For this review, use the dimensioned drawing (mm, ordinates from the lowest corner) and the shaded views. Coordinates: 2 decimals unless noted, no trailing zeros. Loops run counter-clockwise (first coordinate to the right, second up) from the corner with the lowest first, then second, coordinate; pieces in that order, holes last. Notation, with made-up numbers: (-6, 26) -> (7, 26) arc R6 ccw to (7, 37) -> close; hole circle Ø8 at (82.5, 26.25). An arc over 180 degrees is marked (long way). Answer as a JSON object with one key per item and string values.
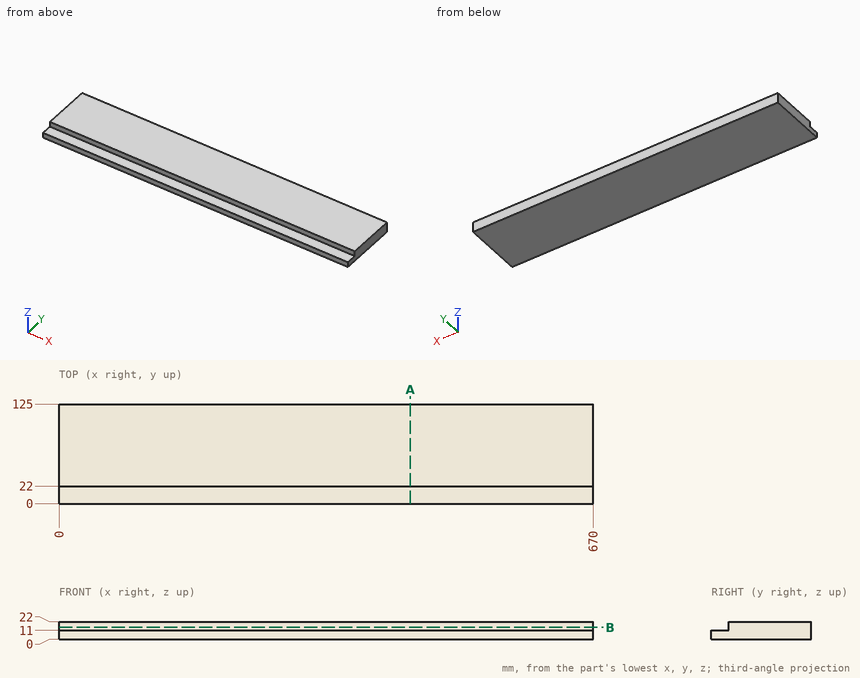
1) Clearance check with a flat-ended pin moving along its axis: pin 1 Ø6.5 at (x, y) = (189, 16) entering from +Z. State where the tip first meets the part, or that it passes through.
Completed:
{"pin 1": "z = 11"}
2) Add section B-B, the plane z = 14.75. Give the boundary of the cut face in (x, y).
Completed:
{"outline": "(0, 22) -> (670, 22) -> (670, 125) -> (0, 125) -> close"}
3) Add section A-A, the plane x = 440.5. Give the boundary of the cut face in (y, z).
Completed:
{"outline": "(0, 0) -> (125, 0) -> (125, 22) -> (22, 22) -> (22, 11) -> (0, 11) -> close"}
4) Wall thickness on probe 1 along Y at (x, z) = (206, 20); probe 2 along Z at (x, y) = (360, 21): over which ranges is each line inside the solid? List them lowest first.
Completed:
{"probe 1": "22 to 125", "probe 2": "0 to 11"}
